Geometry check sheet. Reference: the model listing, model coordinates, mm. A direction names the side the tool comes from. Round coordinates to 2 decimals unless told otherwise and drop trailing zeros. Loops run counter-clockwise (first coordinate to the right, second up) from the corner with the lowest first, then second, coordinate; pieces in that order, holes last. Notation, with made-up numbers: (46.5, 89) -> (85.5, 89) arc R9 cw to (85.5, 105) -> close; hole circle Ø3 at (49, 56). An arc over 180 degrees is marked (long way). Use one line per item in the form item = value.
from build123d import *

# Parameters (mm, degrees)
F0_R     = 50
F0_R_2   = 25
F1_DEPTH = 10


with BuildPart() as f1:
    # F0 (on Front) → F1 (new body)
    with BuildSketch(Plane.XZ):
        Circle(F0_R)
        with BuildLine():
            ThreePointArc((-20.1618326801, 34.5470766199), (-12.360679775, 38.0422606518), (-3.9949968711, 39.8))
            ThreePointArc((-3.9949968711, 39.8), (-0.1000312842, 43.9987490222), (4, 40))
            ThreePointArc((4, 40), (3.9987490222, 39.8999687158), (3.9949968711, 39.8))
            ThreePointArc((3.9949968711, 39.8), (12.360679775, 38.0422606518), (20.1618326801, 34.5470766199))
            ThreePointArc((20.1618326801, 34.5470766199), (24.6519560911, 36.1946274563), (27.5114100917, 32.360679775))
            ThreePointArc((27.5114100917, 32.360679775), (27.2835350395, 31.0298629662), (26.6258734024, 29.8506761323))
            ThreePointArc((26.6258734024, 29.8506761323), (32.360679775, 23.5114100917), (36.6175274229, 16.0983441829))
            ThreePointArc((36.6175274229, 16.0983441829), (40.3117393457, 15.6545326038), (42.0422606518, 12.360679775))
            ThreePointArc((42.0422606518, 12.360679775), (41.2185196533, 9.9293470632), (39.0865712742, 8.4994085693))
            ThreePointArc((39.0865712742, 8.4994085693), (40, 0), (39.0865712742, -8.4994085693))
            ThreePointArc((39.0865712742, -8.4994085693), (41.2185196533, -9.9293470632), (42.0422606518, -12.360679775))
            ThreePointArc((42.0422606518, -12.360679775), (40.3117393457, -15.6545326038), (36.6175274229, -16.0983441829))
            ThreePointArc((36.6175274229, -16.0983441829), (32.360679775, -23.5114100917), (26.6258734024, -29.8506761323))
            ThreePointArc((26.6258734024, -29.8506761323), (27.2835350395, -31.0298629662), (27.5114100917, -32.360679775))
            ThreePointArc((27.5114100917, -32.360679775), (24.6519560911, -36.1946274563), (20.1618326801, -34.5470766199))
            ThreePointArc((20.1618326801, -34.5470766199), (12.360679775, -38.0422606518), (3.9949968711, -39.8))
            ThreePointArc((3.9949968711, -39.8), (3.9987490222, -39.8999687158), (4, -40))
            ThreePointArc((4, -40), (-0.1000312842, -43.9987490222), (-3.9949968711, -39.8))
            ThreePointArc((-3.9949968711, -39.8), (-12.360679775, -38.0422606518), (-20.1618326801, -34.5470766199))
            ThreePointArc((-20.1618326801, -34.5470766199), (-25.8625511009, -35.5967477525), (-26.6258734024, -29.8506761323))
            ThreePointArc((-26.6258734024, -29.8506761323), (-32.360679775, -23.5114100917), (-36.6175274229, -16.0983441829))
            ThreePointArc((-36.6175274229, -16.0983441829), (-41.846486717, -13.5967477525), (-39.0865712742, -8.4994085693))
            ThreePointArc((-39.0865712742, -8.4994085693), (-40, 0), (-39.0865712742, 8.4994085693))
            ThreePointArc((-39.0865712742, 8.4994085693), (-41.846486717, 13.5967477525), (-36.6175274229, 16.0983441829))
            ThreePointArc((-36.6175274229, 16.0983441829), (-32.360679775, 23.5114100917), (-26.6258734024, 29.8506761323))
            ThreePointArc((-26.6258734024, 29.8506761323), (-25.8625511009, 35.5967477525), (-20.1618326801, 34.5470766199))
        make_face(mode=Mode.SUBTRACT)
        with BuildLine():
            ThreePointArc((3.9949968711, 39.8), (0, 36), (-3.9949968711, 39.8))
            ThreePointArc((-3.9949968711, 39.8), (-12.360679775, 38.0422606518), (-20.1618326801, 34.5470766199))
            ThreePointArc((-20.1618326801, 34.5470766199), (-19.6774624104, 33.5012257744), (-19.5114100917, 32.360679775))
            ThreePointArc((-19.5114100917, 32.360679775), (-22.1805932829, 28.5885548272), (-26.6258734024, 29.8506761323))
            ThreePointArc((-26.6258734024, 29.8506761323), (-32.360679775, 23.5114100917), (-36.6175274229, 16.0983441829))
            ThreePointArc((-36.6175274229, 16.0983441829), (-34.748407823, 14.6301584689), (-34.0422606518, 12.360679775))
            ThreePointArc((-34.0422606518, 12.360679775), (-35.6109279401, 9.1844207735), (-39.0865712742, 8.4994085693))
            ThreePointArc((-39.0865712742, 8.4994085693), (-40, 0), (-39.0865712742, -8.4994085693))
            ThreePointArc((-39.0865712742, -8.4994085693), (-35.6109279401, -9.1844207735), (-34.0422606518, -12.360679775))
            ThreePointArc((-34.0422606518, -12.360679775), (-34.748407823, -14.6301584689), (-36.6175274229, -16.0983441829))
            ThreePointArc((-36.6175274229, -16.0983441829), (-32.360679775, -23.5114100917), (-26.6258734024, -29.8506761323))
            ThreePointArc((-26.6258734024, -29.8506761323), (-22.1805932829, -28.5885548272), (-19.5114100917, -32.360679775))
            ThreePointArc((-19.5114100917, -32.360679775), (-19.6774624104, -33.5012257744), (-20.1618326801, -34.5470766199))
            ThreePointArc((-20.1618326801, -34.5470766199), (-12.360679775, -38.0422606518), (-3.9949968711, -39.8))
            ThreePointArc((-3.9949968711, -39.8), (0, -36), (3.9949968711, -39.8))
            ThreePointArc((3.9949968711, -39.8), (12.360679775, -38.0422606518), (20.1618326801, -34.5470766199))
            ThreePointArc((20.1618326801, -34.5470766199), (21.1602690825, -29.1246117975), (26.6258734024, -29.8506761323))
            ThreePointArc((26.6258734024, -29.8506761323), (32.360679775, -23.5114100917), (36.6175274229, -16.0983441829))
            ThreePointArc((36.6175274229, -16.0983441829), (34.2380345866, -11.1246117975), (39.0865712742, -8.4994085693))
            ThreePointArc((39.0865712742, -8.4994085693), (40, 0), (39.0865712742, 8.4994085693))
            ThreePointArc((39.0865712742, 8.4994085693), (34.2380345866, 11.1246117975), (36.6175274229, 16.0983441829))
            ThreePointArc((36.6175274229, 16.0983441829), (32.360679775, 23.5114100917), (26.6258734024, 29.8506761323))
            ThreePointArc((26.6258734024, 29.8506761323), (21.1602690825, 29.1246117975), (20.1618326801, 34.5470766199))
            ThreePointArc((20.1618326801, 34.5470766199), (12.360679775, 38.0422606518), (3.9949968711, 39.8))
        make_face()
        Circle(F0_R_2, mode=Mode.SUBTRACT)
        Circle(F0_R_2)
        with BuildLine():
            ThreePointArc((-13.2287565553, -15), (-20, 0), (-13.2287565553, 15))
            Line((-13.2287565553, 15), (13.2287565553, 15))
            ThreePointArc((13.2287565553, 15), (20, 0), (13.2287565553, -15))
            Line((13.2287565553, -15), (-13.2287565553, -15))
        make_face(mode=Mode.SUBTRACT)
    extrude(amount=F1_DEPTH)


solid = f1.part
1. Gauge pin test, flat ends, axial feed: pin 1 (2 mm diameter, centred on x = -6.5, y = -7.5, fed in from +Z); pin 2 (5 mm diameter, centred on x = -1.5, y = -7, fed in from +Z). Record the tip position at first contact, or that the pin passes through.
Return value:
pin_1 = 49.7
pin_2 = 50
2. Section check D-D (x = -21.5). Record the boundary of the cut face in (y, z).
Return value:
outline = (-10, -45.14) -> (0, -45.14) -> (0, -35.82) -> (-10, -35.82) -> close; (-10, -28.9) -> (0, -28.9) -> (0, 28.9) -> (-10, 28.9) -> close; (-10, 35.82) -> (0, 35.82) -> (0, 45.14) -> (-10, 45.14) -> close
3. Mould release check, pull along X, two halves, no side actions. Record for faces 3 (the cylindrical face through (20, -5, 0)), 4 (the cylindrical face through (47.69, -4.93, 15.02)), 5 (the flat face through (22, 0, 1)): released by +X, released by -X, zero draft, split by the parting line, or undercut.
Return value:
face_3 = undercut
face_4 = split by the parting line
face_5 = zero draft
4. Section check C-C (x = 17). Record the boundary of the cut face in (y, z), then the cut area to 3 significant figures.
Return value:
outline = (-10, -47.02) -> (0, -47.02) -> (0, -10.54) -> (-10, -10.54) -> close; (-10, 10.54) -> (0, 10.54) -> (0, 47.02) -> (-10, 47.02) -> close
area = 730 mm2
5. Material ranges on line 1 along Z through (x, y) = (21.5, -7.25); line 2 along X through (y, z) = (-8, -34); line 3 along Z through (x, y) = (-37, -6.5), recorded low to high.
Return value:
line_1 = -45.14 to -35.82, -28.9 to 28.9, 35.82 to 45.14
line_2 = -36.66 to -27.16, -19.86 to 19.86, 27.16 to 36.66
line_3 = -33.63 to -16.22, -8.5 to 8.5, 16.22 to 33.63
6. Section check B-B (x = 0). Record the boundary of the cut face in (y, z), then the cut area to 3 significant figures.
Return value:
outline = (-10, -50) -> (0, -50) -> (0, -44) -> (-10, -44) -> close; (-10, -36) -> (0, -36) -> (0, -15) -> (-10, -15) -> close; (-10, 15) -> (0, 15) -> (0, 36) -> (-10, 36) -> close; (-10, 44) -> (0, 44) -> (0, 50) -> (-10, 50) -> close
area = 540 mm2
7. Tool access check on faces 1 (the flat face through (22, -10, 1)), 2 (the cylindrical face through (-20, -5, 0)). Record the directions out of +Z, -Z, +X, -X, +Y, -Y that give a thin tool (end or side, any length) a straight path to the whole face; none if there is none.
Return value:
face_1 = +Z, -Z, +X, -X, -Y
face_2 = +Y, -Y
8. Section check A-A (z = 0). Record the boundary of the cut face in (x, y).
Return value:
outline = (-50, -10) -> (-20, -10) -> (-20, 0) -> (-50, 0) -> close; (20, -10) -> (50, -10) -> (50, 0) -> (20, 0) -> close
